Drawing for the job (mm, zero at the part's lowest x, y, z). A direction names the side the tool comes from. Coordinates: 2 decimals unless noted, no trailing zeros. Order: outer loops, then holes, each group sorted by start corner. A loop starts at its lowest first (then second) coordinate and runs counter-clockwise, first axis right, second up. Notation, with made-up numbers: (-23.75, 37.25) -> (2.25, 37.25) arc R17 cw to (2.25, 62.25) -> close; hole circle Ø6 at (60.5, 75.5). An arc over 180 degrees is marked (long way). Write each question's results on one line, items separated by ' | '.
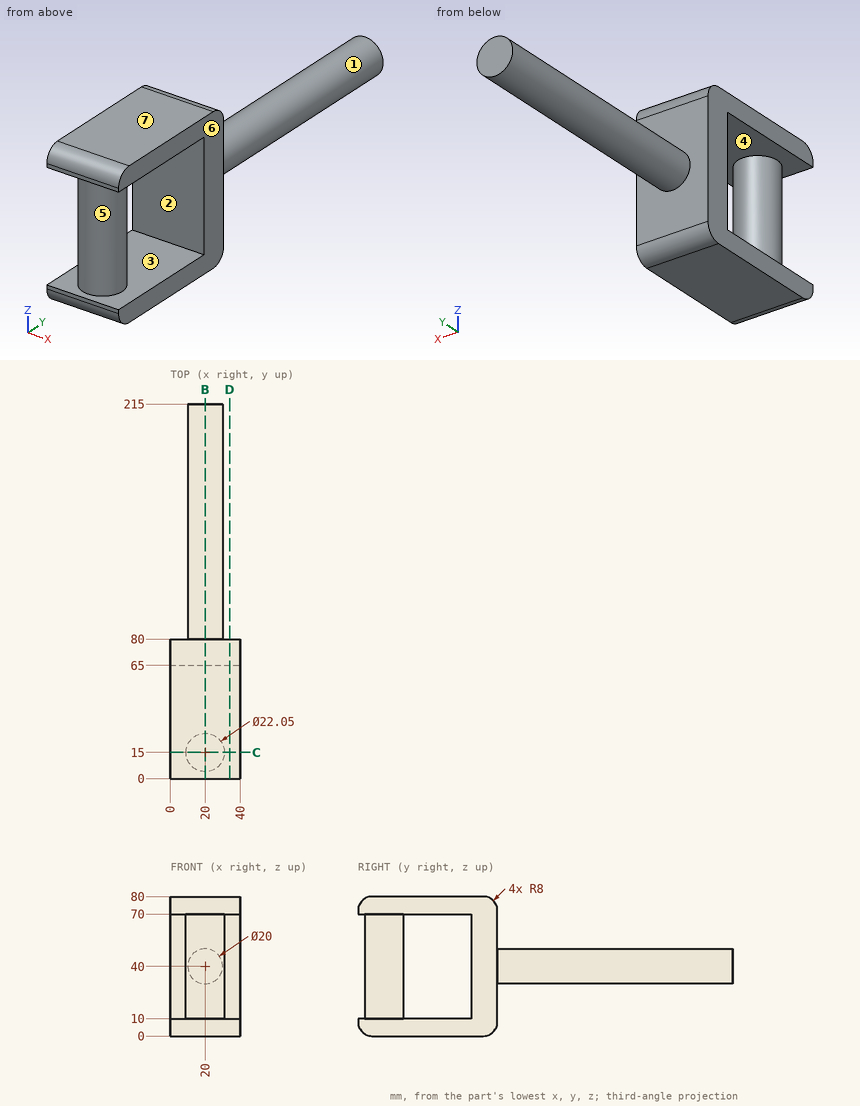
Item 1: Slice it at B-B, the plane x = 20. List the corners of the cut face in (y, z) (1 decimal).
Answer:
outline: (0, 8) arc R8 ccw to (8, 0) -> (72, 0) arc R8 ccw to (80, 8) -> (80, 30) -> (215, 30) -> (215, 50) -> (80, 50) -> (80, 72) arc R8 ccw to (72, 80) -> (8, 80) arc R8 ccw to (0, 72) -> (0, 70) -> (4, 70) -> (4, 10) -> (0, 10) -> close; hole (26, 10) -> (65, 10) -> (65, 70) -> (26, 70) -> close
Item 2: Slice it at C-C, the plane y = 15. List the corners of the cut face in (x, z) (1 decimal).
Answer:
outline: (0, 0) -> (40, 0) -> (40, 10) -> (31, 10) -> (31, 70) -> (40, 70) -> (40, 80) -> (0, 80) -> (0, 70) -> (9, 70) -> (9, 10) -> (0, 10) -> close
Item 3: Pull direction Z, two halves, no side cores. Call the marked faces 4, 5, 6 and 7: released by +Z, released by -Z, zero draft, split by the parting line, or undercut.
Answer:
face 4: undercut | face 5: undercut | face 6: zero draft | face 7: released by +Z
Item 4: Tool access for the marked faces 1, 2 and 3: list every direction of +Z, -Z, +X, -X, +Y, -Y with a clear straight run to the whole face (end or side of a thin tool).
Answer:
face 1: +Y | face 2: +X, -X | face 3: none
Item 5: Slice it at D-D, the plane x = 34. List the corners of the cut face in (y, z), and give its area (4 significant figures).
Answer:
outline: (0, 8) arc R8 ccw to (8, 0) -> (72, 0) arc R8 ccw to (80, 8) -> (80, 72) arc R8 ccw to (72, 80) -> (8, 80) arc R8 ccw to (0, 72) -> (0, 70) -> (65, 70) -> (65, 10) -> (0, 10) -> close | area: 2,445 mm^2
Item 6: Pin check, flat tips, straight feed: pin 1 (5 mm diameter, centred on y = 107.5, z = 51.5, fed in from -X); pin 2 (8 mm diameter, centred on y = 127.5, z = 35, fed in from -X). Stop position of each tip, or through.
Answer:
pin 1: stops at x = 15.64 | pin 2: stops at x = 10.05
Item 7: Drill centre lines: line 1 (Z direction, x = 24.5, y = 50); line 2 (Y direction, x = 20, z = 26) (1 decimal); line 3 (Y direction, x = 38, z = 39). Where is each one in solid material? Low to high. Write a range as from..to.
Answer:
line 1: z = 0..10, 70..80 | line 2: y = 4..26, 65..80 | line 3: y = 65..80
